Can you work these out from the model? Positions are in its coordinate system, mm. A direction names the side the tool comes from. Give positions to 0.01 mm unless a question says otherwise; leave off trailing zeros. Order: outer loops, then holes, each group sorted by start corner. A loop starts at its lowest first (then second) coordinate and runs counter-clockwise, first axis right, second up.
```python
from build123d import *

# Parameters (mm, degrees)
SKETCH1_R           = 18
BOSS_EXTRUDE1_DEPTH = 57
SKETCH2_R           = 17
BOSS_EXTRUDE2_DEPTH = 0.5
SKETCH3_R           = 18
BOSS_EXTRUDE3_DEPTH = 23.5
SKETCH4_R           = 6
SKETCH4_R_2         = 3
BOSS_EXTRUDE4_DEPTH = 6.3
SKETCH6_R           = 1.5
CUT_EXTRUDE1_DEPTH  = 3.5
SKETCH7_R           = 5.5
BOSS_EXTRUDE6_DEPTH = 2
SKETCH8_R           = 1.5
BOSS_EXTRUDE7_DEPTH = 9
SKETCH9_W           = 0.5
SKETCH9_H           = 3.8
BOSS_EXTRUDE8_DEPTH = 7
BOSS_EXTRUDE9_DEPTH = 34


with BuildPart() as part:
    # Sketch1 → Boss-Extrude1 (new body)
    with BuildSketch(Plane(origin=(0, 0, 0), x_dir=(0, 0, -1), z_dir=(1, 0, 0))):
        Circle(SKETCH1_R)
    extrude(amount=BOSS_EXTRUDE1_DEPTH)

    # Sketch2 → Boss-Extrude2 (add)
    with BuildSketch(Plane(origin=(57, 0, 0), x_dir=(0, 0, -1), z_dir=(1, 0, 0))):
        Circle(SKETCH2_R)
    extrude(amount=BOSS_EXTRUDE2_DEPTH)

    # Sketch3 → Boss-Extrude3 (add)
    with BuildSketch(Plane(origin=(57.5, 0, 0), x_dir=(0, 0, -1), z_dir=(1, 0, 0))):
        Circle(SKETCH3_R)
    extrude(amount=BOSS_EXTRUDE3_DEPTH)

    # Sketch4 → Boss-Extrude4 (add)
    with BuildSketch(Plane(origin=(81, 0, 0), x_dir=(0, 0, -1), z_dir=(1, 0, 0))):
        with Locations((0, 7)):
            Circle(SKETCH4_R)
        with Locations((0, 7)):
            Circle(SKETCH4_R_2, mode=Mode.SUBTRACT)
    extrude(amount=BOSS_EXTRUDE4_DEPTH)

    # Sketch6 → Cut-Extrude1 (cut)
    with BuildSketch(Plane(origin=(81, 0, 0), x_dir=(0, 0, -1), z_dir=(1, 0, 0))):
        with Locations((-15.5, 0)):
            Circle(SKETCH6_R)
        with Locations((-7.75, 13.423393759)):
            Circle(SKETCH6_R)
        with Locations((7.75, 13.423393759)):
            Circle(SKETCH6_R)
        with Locations((15.5, 0)):
            Circle(SKETCH6_R)
        with Locations((7.75, -13.423393759)):
            Circle(SKETCH6_R)
        with Locations((-7.75, -13.423393759)):
            Circle(SKETCH6_R)
    extrude(amount=-CUT_EXTRUDE1_DEPTH, mode=Mode.SUBTRACT)

    # Sketch7 → Boss-Extrude6 (add)
    with BuildSketch(Plane.ZY):
        Circle(SKETCH7_R)
    extrude(amount=BOSS_EXTRUDE6_DEPTH)

    # Sketch8 → Boss-Extrude7 (add)
    with BuildSketch(Plane.ZY.offset(2)):
        Circle(SKETCH8_R)
    extrude(amount=BOSS_EXTRUDE7_DEPTH)

    # Sketch9 → Boss-Extrude8 (add)
    with BuildSketch(Plane.ZY):
        with Locations((13.5, 0)):
            Rectangle(SKETCH9_W, SKETCH9_H)
        with Locations((-13.434451739, 0)):
            Rectangle(SKETCH9_W, SKETCH9_H)
    extrude(amount=BOSS_EXTRUDE8_DEPTH)

    # Sketch10 → Boss-Extrude9 (add)
    with BuildSketch(Plane(origin=(54, 0, 0), x_dir=(0, 0, -1), z_dir=(1, 0, 0))):
        with BuildLine():
            Line((2.881280854, -17.767898599), (2.961316433, -18.261451338))
            ThreePointArc((2.961316433, -18.261451338), (0, 18.5), (-2.961316433, -18.261451338))
            Line((-2.961316433, -18.261451338), (-2.881280854, -17.767898599))
            ThreePointArc((-2.881280854, -17.767898599), (0, 18), (2.881280854, -17.767898599))
        make_face()
    extrude(amount=-BOSS_EXTRUDE9_DEPTH)


solid = part.part
```
1) Suppose I cut it at D-D (z = 15.5). Please give me the cut outline in (x, y).
2) Which directions (+Z, -Z, +X, -X, +Y, -Y) give clear straight access to the entire face, cutting with the end or side of a thin tool? Please do faces 5 (the face through (-3, 0, -13.184)), 6 (the face through (-2, -1.1, -1.3)), 7 (the face through (77.5, -13, 8)), 8 (the face through (-3, 0, -13.684)).
3) I'm going to push flat-ended pins straight in: pin 1 Ø5 at (x, z) = (57.5, 5.5) entering from +Y; pin 2 Ø3 at (y, z) = (8, 1) entering from +X; pin 3 Ø18 at (y, z) = (8.5, -7) entering from -X. Where does each tip first touch, or does it pass through?
4) We'd pull the mould along Z, two halves only. Please class faces 1 (the face through (87.3, 10, -1)), 2 (the face through (-6.44, 0.07, -1.5)), 3 (the face through (57.246, 14.334, -9.139)), 4 (the face through (79.274, -12.41, -6.644)): +Z half, -Z half, draft (parallel to the pull), parting line (faces both ways), or undercut.
5) If I drill on line 1 (Y direction, x = 79.95, z = -7.75); line 2 (X direction, y = -13, z = -12); line 3 (X direction, y = 3, z = -2.5), over which ranges is the centre line in solid material (lowest first)?
6) Suppose I cut it at C-C (x = 29.5). Please give me the cut outline in (y, z), and give its area (3 significant figures).
7) Suppose I cut it at A-A (x = 79.5). Please give me the cut outline in (y, z), and give its area (3 significant figures).
Results:
1. outline: (0, -9.15) - (20, -9.15) - (20, -10.1) - (54, -10.1) - (54, -9.15) - (57, -9.15) - (57, -6.98) - (57.5, -6.98) - (57.5, -9.15) - (81, -9.15) - (81, -1.5) - (77.5, -1.5) - (77.5, 1.5) - (81, 1.5) - (81, 9.15) - (57.5, 9.15) - (57.5, 6.98) - (57, 6.98) - (57, 9.15) - (54, 9.15) - (54, 10.1) - (20, 10.1) - (20, 9.15) - (0, 9.15) - close
2. face 5: -X, +Y, -Y
2. face 6: -X
2. face 7: +X
2. face 8: -Z, -X, +Y, -Y
3. pin 1: stops at y = 17.75
3. pin 2: stops at x = 81
3. pin 3: stops at x = -2
4. face 1: draft
4. face 2: undercut
4. face 3: parting line
4. face 4: undercut
5. line 1: y = -16.25 to -14.92, -11.92 to 11.92, 14.92 to 16.25
5. line 2: x = 0 to 57, 57.5 to 81
5. line 3: x = -2 to 87.3
6. outline: (-18.26, -2.96) arc R18.5 ccw (long way) to (-18.26, 2.96) - (-17.77, 2.88) arc R18 ccw to (-17.77, -2.88) - close
6. area: 1,070 mm2
7. outline: circle Ø36 at (0, 0); hole circle Ø3 at (-13.42, -7.75); hole circle Ø3 at (-13.42, 7.75); hole circle Ø3 at (0, -15.5); hole circle Ø3 at (0, 15.5); hole circle Ø3 at (13.42, -7.75); hole circle Ø3 at (13.42, 7.75)
7. area: 975 mm2
